Geometry check sheet. Reference: the model listing, model coordinates, mm. Round coordinates to 2 decimals unless told otherwise and drop trailing zeros. Write each loop counter-clockwise with the first axis right and the second up, starting at its lowest first coordinate (ties: lowest second). Pieces come first, ordered by that corner, then holes. Notation, with made-up numbers: (58.25, -28) -> (71.25, -28) arc R24 cw to (71.25, -1) -> close; hole circle Ø9 at (-32.75, 54). An arc over 180 degrees is marked (long way). Put each result on its own line as item: value. Start each with the question number.
from build123d import *

# Parameters (mm, degrees)
F0_W      = 190.5
F0_H      = 190.5
F0_R      = 3.175
F1_DEPTH  = 6.35
F3_DEPTH  = 6.351
F5_DEPTH  = 6.351
F6_R      = 5.715
F7_DEPTH  = 6.351
F8_R      = 3.175
F8_R_2    = 19.05
F9_DEPTH  = 6.351
F10_R     = 12.7
F12_DEPTH = 6.351
F13_R     = 13.843
F14_DEPTH = 6.351


with BuildPart() as f1:
    # F0 (on Top) → F1 (new body)
    with BuildSketch(Plane.XY):
        Rectangle(F0_W, F0_H)
        with Locations((-82.55, -82.55)):
            Circle(F0_R, mode=Mode.SUBTRACT)
        with Locations((82.55, -82.55)):
            Circle(F0_R, mode=Mode.SUBTRACT)
        with Locations((-82.55, 82.55)):
            Circle(F0_R, mode=Mode.SUBTRACT)
        with Locations((82.55, 82.55)):
            Circle(F0_R, mode=Mode.SUBTRACT)
    extrude(amount=F1_DEPTH)

    # F2 (on face) → F3 (cut, through all)
    with BuildSketch(Plane.XY.offset(6.35)):
        with BuildLine():
            Line((-88.9, 61.4426), (-88.9, 63.5))
            Line((-88.9, 63.5), (-86.8426, 63.5))
            ThreePointArc((-86.8426, 63.5), (-90.354801, 64.954801), (-88.9, 61.4426))
        make_face()
        with BuildLine():
            Line((-86.8426, 63.5), (-88.9, 63.5))
            Line((-88.9, 63.5), (-88.9, 61.4426))
            ThreePointArc((-88.9, 61.4426), (-87.445199, 62.045199), (-86.8426, 63.5))
        make_face()
        with BuildLine():
            Line((-57.15, 63.5), (-59.2074, 63.5))
            ThreePointArc((-59.2074, 63.5), (-58.604801, 62.045199), (-57.15, 61.4426))
            Line((-57.15, 61.4426), (-57.15, 63.5))
        make_face()
        with BuildLine():
            ThreePointArc((-55.0926, 63.5), (-57.15, 65.5574), (-59.2074, 63.5))
            Line((-59.2074, 63.5), (-57.15, 63.5))
            Line((-57.15, 63.5), (-57.15, 61.4426))
            ThreePointArc((-57.15, 61.4426), (-55.695199, 62.045199), (-55.0926, 63.5))
        make_face()
        with BuildLine():
            ThreePointArc((-86.8426, 25.4), (-87.445199, 26.854801), (-88.9, 27.4574))
            Line((-88.9, 27.4574), (-88.9, 25.4))
            Line((-88.9, 25.4), (-86.8426, 25.4))
        make_face()
        with BuildLine():
            Line((-88.9, 25.4), (-88.9, 27.4574))
            ThreePointArc((-88.9, 27.4574), (-90.354801, 23.945199), (-86.8426, 25.4))
            Line((-86.8426, 25.4), (-88.9, 25.4))
        make_face()
        with BuildLine():
            Line((-57.15, 25.4), (-57.15, 27.4574))
            ThreePointArc((-57.15, 27.4574), (-58.604801, 26.854801), (-59.2074, 25.4))
            Line((-59.2074, 25.4), (-57.15, 25.4))
        make_face()
        with BuildLine():
            ThreePointArc((-55.0926, 25.4), (-55.695199, 26.854801), (-57.15, 27.4574))
            Line((-57.15, 27.4574), (-57.15, 25.4))
            Line((-57.15, 25.4), (-59.2074, 25.4))
            ThreePointArc((-59.2074, 25.4), (-57.15, 23.3426), (-55.0926, 25.4))
        make_face()
    extrude(amount=-F3_DEPTH, mode=Mode.SUBTRACT)

    # F4 (on face) → F5 (cut, through all)
    with BuildSketch(Plane.XY.offset(6.35)):
        with BuildLine():
            Line((-44.45, -42.3926), (-44.45, -44.45))
            Line((-44.45, -44.45), (-42.3926, -44.45))
            ThreePointArc((-42.3926, -44.45), (-42.995199, -42.995199), (-44.45, -42.3926))
        make_face()
        with BuildLine():
            Line((-42.3926, -44.45), (-44.45, -44.45))
            Line((-44.45, -44.45), (-44.45, -42.3926))
            ThreePointArc((-44.45, -42.3926), (-45.904801, -45.904801), (-42.3926, -44.45))
        make_face()
        with BuildLine():
            ThreePointArc((44.45, -42.3926), (42.995199, -42.995199), (42.3926, -44.45))
            Line((42.3926, -44.45), (44.45, -44.45))
            Line((44.45, -44.45), (44.45, -42.3926))
        make_face()
        with BuildLine():
            Line((44.45, -44.45), (42.3926, -44.45))
            ThreePointArc((42.3926, -44.45), (44.45, -46.5074), (46.5074, -44.45))
            ThreePointArc((46.5074, -44.45), (45.904801, -42.995199), (44.45, -42.3926))
            Line((44.45, -42.3926), (44.45, -44.45))
        make_face()
        with BuildLine():
            ThreePointArc((-42.3926, 44.45), (-45.904801, 45.904801), (-44.45, 42.3926))
            Line((-44.45, 42.3926), (-44.45, 44.45))
            Line((-44.45, 44.45), (-42.3926, 44.45))
        make_face()
        with BuildLine():
            Line((-44.45, 44.45), (-44.45, 42.3926))
            ThreePointArc((-44.45, 42.3926), (-42.995199, 42.995199), (-42.3926, 44.45))
            Line((-42.3926, 44.45), (-44.45, 44.45))
        make_face()
        with BuildLine():
            ThreePointArc((42.3926, 44.45), (42.995199, 42.995199), (44.45, 42.3926))
            Line((44.45, 42.3926), (44.45, 44.45))
            Line((44.45, 44.45), (42.3926, 44.45))
        make_face()
        with BuildLine():
            Line((44.45, 44.45), (44.45, 42.3926))
            ThreePointArc((44.45, 42.3926), (45.904801, 42.995199), (46.5074, 44.45))
            ThreePointArc((46.5074, 44.45), (44.45, 46.5074), (42.3926, 44.45))
            Line((42.3926, 44.45), (44.45, 44.45))
        make_face()
    extrude(amount=-F5_DEPTH, mode=Mode.SUBTRACT)

    # F6 (on face) → F7 (cut, through all)
    with BuildSketch(Plane.XY.offset(6.35)):
        with Locations((77.7875, 57.15)):
            Circle(F6_R)
    extrude(amount=-F7_DEPTH, mode=Mode.SUBTRACT)

    # F8 (on face) → F9 (cut, through all)
    with BuildSketch(Plane.XY.offset(6.35)):
        with Locations((-33.3375, -34.925)):
            Circle(F8_R)
        with Locations((33.3375, -34.925)):
            Circle(F8_R)
        with Locations((0, 32.385)):
            Circle(F8_R)
        Circle(F8_R_2)
    extrude(amount=-F9_DEPTH, mode=Mode.SUBTRACT)

    # F10
    f10_edges = [f1.edges().sort_by_distance(p)[0] for p in [
        (-95.25, 95.25, 3.175),
        (95.25, 95.25, 3.175),
        (95.25, -95.25, 3.175),
        (-95.25, -95.25, 3.175),
    ]]
    fillet(f10_edges, radius=F10_R)

    # F11 (on face) → F12 (cut, through all)
    with BuildSketch(Plane.XY.offset(6.35)):
        with BuildLine():
            Line((0, 81.2038), (0, 82.55))
            Line((0, 82.55), (1.3462, 82.55))
            ThreePointArc((1.3462, 82.55), (-0.951907, 83.501907), (0, 81.2038))
        make_face()
        with BuildLine():
            ThreePointArc((26.7462, 82.55), (25.4, 83.8962), (24.0538, 82.55))
            Line((24.0538, 82.55), (25.4, 82.55))
            Line((25.4, 82.55), (25.4, 81.2038))
            ThreePointArc((25.4, 81.2038), (26.351907, 81.598093), (26.7462, 82.55))
        make_face()
        with BuildLine():
            ThreePointArc((26.7462, 57.15), (26.351907, 58.101907), (25.4, 58.4962))
            Line((25.4, 58.4962), (25.4, 57.15))
            Line((25.4, 57.15), (24.0538, 57.15))
            ThreePointArc((24.0538, 57.15), (25.4, 55.8038), (26.7462, 57.15))
        make_face()
        with BuildLine():
            Line((25.4, 82.55), (24.0538, 82.55))
            ThreePointArc((24.0538, 82.55), (24.448093, 81.598093), (25.4, 81.2038))
            Line((25.4, 81.2038), (25.4, 82.55))
        make_face()
        with BuildLine():
            Line((25.4, 57.15), (25.4, 58.4962))
            ThreePointArc((25.4, 58.4962), (24.448093, 58.101907), (24.0538, 57.15))
            Line((24.0538, 57.15), (25.4, 57.15))
        make_face()
        with BuildLine():
            ThreePointArc((1.3462, 57.15), (0.951907, 58.101907), (0, 58.4962))
            Line((0, 58.4962), (0, 57.15))
            Line((0, 57.15), (1.3462, 57.15))
        make_face()
        with BuildLine():
            Line((0, 57.15), (0, 58.4962))
            ThreePointArc((0, 58.4962), (-0.951907, 56.198093), (1.3462, 57.15))
            Line((1.3462, 57.15), (0, 57.15))
        make_face()
        with BuildLine():
            Line((1.3462, 82.55), (0, 82.55))
            Line((0, 82.55), (0, 81.2038))
            ThreePointArc((0, 81.2038), (0.951907, 81.598093), (1.3462, 82.55))
        make_face()
    extrude(amount=-F12_DEPTH, mode=Mode.SUBTRACT)

    # F13 (on face) → F14 (cut, through all)
    with BuildSketch(Plane.XY.offset(6.35)):
        with Locations((-72.39, 0)):
            Circle(F13_R)
        with Locations((72.39, 0)):
            Circle(F13_R)
    extrude(amount=-F14_DEPTH, mode=Mode.SUBTRACT)


solid = f1.part
(1) Sectioned sample at B-B (x = -10.5). Record the cut outline in (y, z).
(2) Material ranges on L1, parallel to X at y = -44.45, z = 4.25; L2, parallel to X at y = 7.5, z = 3; L3, parallel to X at y = -5.5, z = 4.25, recorded low to high. Write a range as from..to.
(3) Mould release check, pull along X, two halves, no side actions. Record for faces 1 (the flat face through (-95.25, -1, 3)), 2 (the cylindrical face through (84.015, 79.733, 3.131)), 3 (the cylindrical face through (1.71, 35.06, 3.22)), 4 (the flat face through (-1, -95.25, 3)): +X half, -X half, draft (parallel to the pull), parting line (faces both ways), or undercut.
(4) Go/stop test with a flat-tipped pin: pin 1 Ø3.5 at (x, y) = (-44.45, 44.45) entering from +Z. Record where the tip stops, or that it passes through.
(5) Sectioned sample at C-C (z = 1.5). State how many separate pieces and enclosed holes the cut face has, and give its area (3 significant figures).
(6) Sectioned sample at A-A (y = 0). Record the cut outline in (x, z), and give its area (3 significant figures).
Found:
1. outline: (-95.25, 0) -> (-15.9, 0) -> (-15.9, 6.35) -> (-95.25, 6.35) -> close; (15.9, 0) -> (95.25, 0) -> (95.25, 6.35) -> (15.9, 6.35) -> close
2. L1: -95.25..-46.51, -42.39..42.39, 46.51..95.25
2. L2: -95.25..-84.03, -60.75..-17.51, 17.51..60.75, 84.03..95.25
2. L3: -95.25..-85.09, -59.69..-18.24, 18.24..59.69, 85.09..95.25
3. face 1: -X half
3. face 2: undercut
3. face 3: undercut
3. face 4: draft
4. pin 1: through
5. separate pieces: 1
5. enclosed holes: 23
5. area: 33,400 mm2
6. outline: (-95.25, 0) -> (-86.23, 0) -> (-86.23, 6.35) -> (-95.25, 6.35) -> close; (-58.55, 0) -> (-19.05, 0) -> (-19.05, 6.35) -> (-58.55, 6.35) -> close; (19.05, 0) -> (58.55, 0) -> (58.55, 6.35) -> (19.05, 6.35) -> close; (86.23, 0) -> (95.25, 0) -> (95.25, 6.35) -> (86.23, 6.35) -> close
6. area: 616 mm2
